Can you work these out from the model? Positions are in its coordinate system, mm. Face numbers are marked on the shaded views. A direction names the side the tool comes from. Round coordinates to 2 decimals unless told otherwise and drop trailing zeros. Loops run counter-clockwise (first coordinate to the right, second up) from the corner with the lowest first, then second, coordinate; pieces in that order, holes last.
Autodesk Inventor part; units mm, degrees
ref_plane "YZ Plane" through (0, 0, 0) normal (1, 0, 0) x (0, 1, 0)
ref_plane "XZ Plane" through (0, 0, 0) normal (0, 1, 0) x (-1, 0, 0)
ref_plane "XY Plane" through (0, 0, 0) normal (0, 0, 1) x (1, 0, 0)
sketch "Sketch1" plane through (0, 0, 0) normal (0, 1, 0) x (-1, 0, 0)
  circle A0 centre (0, 0) radius 25
  circle A1 centre (0, 0) radius 26.6
  line L0 (25, 1) -> (25, 0)
  line L1 (25, 0) -> (25, -1)
  line L2 (25, -1) -> (21, 0)
  line L3 (21, 0) -> (25, 1)
  line L4 (-25, 0) -> (-25, -1)
  line L5 (-25, -1) -> (-21, 0)
  line L6 (-21, 0) -> (-25, 1)
  line L7 (-25, 1) -> (-25, 0)
  point P0 (24.9802, -0.995)
  point P1 (-24.9802, -0.995)
  point P2 (-24.9802, 0.995)
  point P3 (24.9802, 0.995)
  dimension "d0" = 50
  dimension "d1" = 4
  dimension "d2" = 1
  dimension "d3" = 1
  dimension "d4" = 1.6
  dimension "d5" = 1
  dimension "d6" = 1
  dimension "d7" = 4
extrude "Extrusion1" add sketch "Sketch1" along normal blind 70 contours A0 L2 L3 | L1 L2 A0 | A0 L3 L0 | L6 L5 A0 | A0 L7 L6 | L5 L4 A0 | A1
sketch "Sketch2" plane through (0, 0, 0) normal (0, 0, 1) x (1, 0, 0)
  line L0 (26.6, 0) -> (-26.6, 0)
  line L1 (0.0198, -6.0198) -> (0.0198, -5)
  line L2 (-24.9802, 0) -> (-21, 0)
  line L3 (0.0198, -5) -> (-24.9802, 0)
  line L4 (-24.9802, 0) -> (24.9802, 0)
  line L5 (-24.9802, 0) -> (-26.6, 0)
  line L6 (-26.6, 0) -> (-26.6, -0.6958)
  line L7 (-26.6, -0.6958) -> (0.0198, -6.0198)
  line L8 (0.0198, -6.0198) -> (0.0198, -26.0198)
  line L9 (0.0198, -26.0198) -> (-4.5302, -26.0198)
  line L10 (-4.5302, -26.0198) -> (-4.5302, -5.1098)
  point P0 (0, 0)
  dimension "d16" = 5
  dimension "d19" = 25
  dimension "d20" = 1
  dimension "d22" = 4.55
  dimension "d23" = 20
revolve "Revolution1" add sketch "Sketch2" angle 360 about axis through (0.0198, -6.0198, 0) along (0, 1, 0)
sketch "Sketch4" plane through (0.0198, -26.0198, 0) normal (0, -1, 0) x (1, 0, 0)
  circle A0 centre (-0.0198, 0) radius 2
  dimension "d24" = 4
extrude "Extrusion3" cut sketch "Sketch4" against normal through all
thread "Thread1"
properties part number "Reactor"
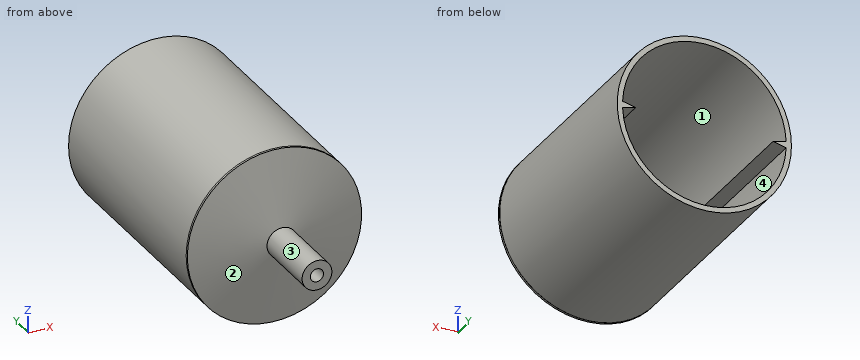
(1) If we section it at A-A, the plane y = 33: List the corners of the cut face in (x, z) for me.
Worked answers:
outline: circle Ø53.2 at (0, 0); hole (-24.98, -1) arc R25 ccw to (24.98, -1) - (21, 0) - (24.98, 1) arc R25 ccw to (-24.98, 1) - (-21, 0) - close
(2) If we mould it in two halves opening along Z, with no side actions, what happens to the marked faces 1 and 2? For each: released by +Z, released by -Z, zero draft, split by the parting line, or undercut.
Worked answers:
face 1: undercut
face 2: split by the parting line
(3) For the marked faces 3 and 4, which set-ups out of +Z, -Z, +X, -X, +Y, -Y let a thin tool reach every point of the face, with its end or its side?
Worked answers:
face 3: -Y
face 4: +Y
(4) If I drill on line 1 (Z direction, x = 0, y = -18); line 2 (X direction, y = 1.5, z = -3.5); line 3 (X direction, y = 52, z = 4), over which ranges is the centre line in solid material (lowest first)?
Worked answers:
line 1: z = -4.55 to -2, 2 to 4.55
line 2: x = -26.37 to -24.75, 24.75 to 26.37
line 3: x = -26.3 to -24.68, 24.68 to 26.3
(5) Will these pins go through, and if not, where does the flat tip stop? P1, Ø12.5, axis at x = 17.5, z = -2, coming from the -Y side; P2, Ø2, axis at x = -23, z = 0, coming from the -Y side; P3, Ø10, axis at x = 10, z = 8.5, coming from the +Y side; P4, Ø12, axis at x = -9.5, z = -17, coming from the +Y side.
Worked answers:
P1: stops at y = -3.75
P2: stops at y = -1.62
P3: stops at y = -1.38
P4: stops at y = 70
